```python
from build123d import *

# Parameters (mm, degrees)
BOSS_EXTRUDE1_DEPTH        = 15
FILLET1_R                  = 30
SKETCH4_R                  = 10
CUT_EXTRUDE1_DEPTH         = 5
M10_CLEARANCE_HOLE1_D      = 11
SKETCH7_R                  = 19.05
CUT_EXTRUDE2_DEPTH         = 16
M4_TAPPED_HOLE1_D          = 3.3
CIRPATTERN2_COUNT          = 3
CIRPATTERN3_COUNT          = 3
M12_CLEARANCE_HOLE1_D      = 13
CIRPATTERN4_COUNT          = 3
F_15_0_15_DIAMETER_HOLE1_D = 15
CIRPATTERN5_COUNT          = 3
F_15_0_15_DIAMETER_HOLE2_D = 15
F_9_0_9_DIAMETER_HOLE1_D   = 9


with BuildPart() as part:
    # Sketch1 → Boss-Extrude1 (new body)
    with BuildSketch(Plane(origin=(0, 0, 0), x_dir=(1, 0, 0), z_dir=(0, 1, 0))):
        with BuildLine():
            ThreePointArc((45, 163.935963108), (0, 170), (-45, 163.935963108))
            Line((-45, 163.935963108), (-45, 77.942286341))
            ThreePointArc((-45, 77.942286341), (-77.942286341, 45), (-90, 0))
            Line((-90, 0), (-164.472708645, -42.996838383))
            ThreePointArc((-164.472708645, -42.996838383), (-147.224318643, -85), (-119.472708645, -120.939124724))
            Line((-119.472708645, -120.939124724), (-45, -77.942286341))
            ThreePointArc((-45, -77.942286341), (0, -90), (45, -77.942286341))
            Line((45, -77.942286341), (119.472708645, -120.939124724))
            ThreePointArc((119.472708645, -120.939124724), (147.224318643, -85), (164.472708645, -42.996838383))
            Line((164.472708645, -42.996838383), (90, 0))
            ThreePointArc((90, 0), (77.942286341, 45), (45, 77.942286341))
            Line((45, 77.942286341), (45, 163.935963108))
        make_face()
    extrude(amount=BOSS_EXTRUDE1_DEPTH)

    # Fillet1
    fillet1_edges = [part.edges().sort_by_distance(p)[0] for p in [
        (-119.472708645, 7.5, 120.939124724),
        (-164.472708645, 7.5, 42.996838383),
        (-90, 7.5, 0),
        (-45, 7.5, -77.942286341),
        (-45, 7.5, -163.935963108),
        (45, 7.5, -163.935963108),
        (45, 7.5, -77.942286341),
        (90, 7.5, 0),
        (164.472708645, 7.5, 42.996838383),
        (119.472708645, 7.5, 120.939124724),
        (45, 7.5, 77.942286341),
        (-45, 7.5, 77.942286341),
    ]]
    fillet(fillet1_edges, radius=FILLET1_R)

    # Sketch4 → Cut-Extrude1 (cut)
    with BuildSketch(Plane(origin=(0, 15, 0), x_dir=(1, 0, 0), z_dir=(0, 1, 0))):
        with Locations((0, 148.5)):
            Circle(SKETCH4_R)
    cut_extrude1 = extrude(amount=-CUT_EXTRUDE1_DEPTH, mode=Mode.SUBTRACT)

    # M10 Clearance Hole1 (through all)
    with Locations(Plane(origin=(0, 15, 0), x_dir=(-1, 0, 0), z_dir=(0, 1, 0))):
        with Locations((0, -148.5)):
            m10_clearance_hole1 = Hole(M10_CLEARANCE_HOLE1_D / 2)

    # Sketch7 → Cut-Extrude2 (cut, through all)
    with BuildSketch(Plane(origin=(0, 15, 0), x_dir=(1, 0, 0), z_dir=(0, 1, 0))):
        with Locations((0, 80)):
            Circle(SKETCH7_R)
    cut_extrude2 = extrude(amount=-CUT_EXTRUDE2_DEPTH, mode=Mode.SUBTRACT)

    # M4 Tapped Hole1 (through all)
    with Locations(Plane(origin=(0, 15, 0), x_dir=(1, 0, 0), z_dir=(0, 1, 0))):
        with Locations((-23.57, 103.57), (23.57, 56.43), (23.57, 103.57), (-23.57, 56.43)):
            m4_tapped_hole1 = Hole(M4_TAPPED_HOLE1_D / 2)

    # CirPattern2: Cut-Extrude2, M4 Tapped Hole1 ×3 about axis
    cirpattern2_axis = Axis((0, 0, 0), (0, 1, 0))
    for i in range(1, CIRPATTERN2_COUNT):
        add(cut_extrude2.rotate(cirpattern2_axis, i * 360 / CIRPATTERN2_COUNT), mode=Mode.SUBTRACT)
        add(m4_tapped_hole1.rotate(cirpattern2_axis, i * 360 / CIRPATTERN2_COUNT), mode=Mode.SUBTRACT)

    # CirPattern3: Cut-Extrude1, M10 Clearance Hole1 ×3 about axis
    cirpattern3_axis = Axis((0, 0, 0), (0, 1, 0))
    for i in range(1, CIRPATTERN3_COUNT):
        add(cut_extrude1.rotate(cirpattern3_axis, i * 360 / CIRPATTERN3_COUNT), mode=Mode.SUBTRACT)
        add(m10_clearance_hole1.rotate(cirpattern3_axis, i * 360 / CIRPATTERN3_COUNT), mode=Mode.SUBTRACT)

    # M12 Clearance Hole1 (through all)
    with Locations(Plane(origin=(0, 15, 0), x_dir=(1, 0, 0), z_dir=(0, 1, 0))):
        with Locations((-39.17442065, -65.983537492)):
            m12_clearance_hole1 = Hole(M12_CLEARANCE_HOLE1_D / 2)

    # CirPattern4: M12 Clearance Hole1 ×3 about axis
    cirpattern4_axis = Axis((0, 0, 0), (0, 1, 0))
    for i in range(1, CIRPATTERN4_COUNT):
        add(m12_clearance_hole1.rotate(cirpattern4_axis, i * 360 / CIRPATTERN4_COUNT), mode=Mode.SUBTRACT)

    # Ø15.0 (15) Diameter Hole1 (through all)
    with Locations(Plane(origin=(0, 0, 0), x_dir=(-1, 0, 0), z_dir=(0, -1, 0))):
        with Locations((0, -70)):
            f_15_0_15_diameter_hole1 = Hole(F_15_0_15_DIAMETER_HOLE1_D / 2)

    # CirPattern5: Ø15.0 (15) Diameter Hole1 ×3 about axis
    cirpattern5_axis = Axis((0, 0, 0), (0, 1, 0))
    for i in range(1, CIRPATTERN5_COUNT):
        add(f_15_0_15_diameter_hole1.rotate(cirpattern5_axis, i * 360 / CIRPATTERN5_COUNT), mode=Mode.SUBTRACT)

    # Ø15.0 (15) Diameter Hole2 (through all)
    with Locations(Plane(origin=(0, 0, 0), x_dir=(-1, 0, 0), z_dir=(0, -1, 0))):
        with Locations((0, 0)):
            Hole(F_15_0_15_DIAMETER_HOLE2_D / 2)

    # Ø9.0 (9) Diameter Hole1 (through all)
    with Locations(Plane(origin=(0, 0, 0), x_dir=(-1, 0, 0), z_dir=(0, -1, 0))):
        with Locations((34.641016151, -20)):
            Hole(F_9_0_9_DIAMETER_HOLE1_D / 2)


solid = part.part
```
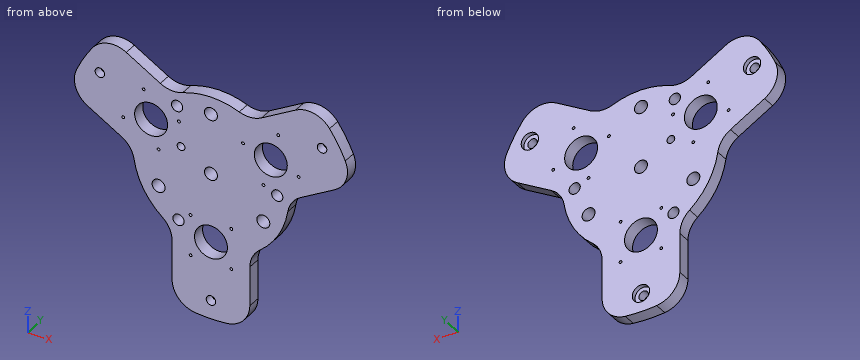
Can you work these out from the model? Positions are in its coordinate system, mm. Coordinates: 2 decimals unless noted, no trailing zeros. Loops run counter-clockwise (first coordinate to the right, second up) from the corner with the lowest first, then second, coordinate; pieces in that order, holes last. Notation, with made-up numbers: (-27, 24.25) - (23, 24.25) arc R14 cw to (23, 42.25) - close; hole circle Ø8 at (41, 60). An arc over 180 degrees is marked (long way). Use a Markdown table: item, result.
Item 1: If I drill on probe 1 along Z at (x, y) = (0, 5); probe 2 along X at (y, z) = (11.5, -39); probe 3 along X at (y, z) = (11.25, 40.5), over which ranges is the centre line in solid material (lowest first)? Write a range as from..to.
Numbers:
| item | result |
|---|---|
| probe 1 | z = -170..-154, -143..-99.05, -60.95..-7.5, 7.5..62.5, 77.5..90 |
| probe 2 | x = -81.11..-66.97, -54.28..54.28, 66.97..81.11 |
| probe 3 | x = -153.36..-88.33, -50.24..50.24, 88.33..153.36 |
Item 2: Will these pins go through, and if not, where does the flat tip stop? pin 1 (7.5 mm diameter, centred on y = 10, z = -109.5, fed in from +X); pin 2 (5 mm diameter, centred on y = 5.5, z = -135.5, fed in from -X); pin 3 (18 mm diameter, centred on x = 0, z = -148.5, fed in from +Y).
Numbers:
| item | result |
|---|---|
| pin 1 | stops at x = 45 |
| pin 2 | stops at x = -45 |
| pin 3 | stops at y = 10 |
Item 3: I want a section at B-B on z = -80. Please give me the cut outline in (x, y).
Numbers:
| item | result |
|---|---|
| outline | (-48.3, 0) - (-19.05, 0) - (-19.05, 15) - (-48.3, 15) - close; (19.05, 0) - (48.3, 0) - (48.3, 15) - (19.05, 15) - close |
Item 4: I want a section at C-C on z = -35. Please give me the cut outline in (x, y), and give its area (3 significant figures).
Numbers:
| item | result |
|---|---|
| outline | (-82.92, 0) - (-68.12, 0) - (-68.12, 15) - (-82.92, 15) - close; (-53.12, 0) - (53.12, 0) - (53.12, 15) - (-53.12, 15) - close; (68.12, 0) - (82.92, 0) - (82.92, 15) - (68.12, 15) - close |
| area | 2,040 mm2 |
Item 5: I want a section at A-A on x = 0. Please give me the cut outline in (y, z), and give its area (3 significant figures).
Numbers:
| item | result |
|---|---|
| outline | (0, -170) - (15, -170) - (15, -158.5) - (10, -158.5) - (10, -154) - (0, -154) - close; (0, -143) - (10, -143) - (10, -138.5) - (15, -138.5) - (15, -99.05) - (0, -99.05) - close; (0, -60.95) - (15, -60.95) - (15, -7.5) - (0, -7.5) - close; (0, 7.5) - (15, 7.5) - (15, 62.5) - (0, 62.5) - close; (0, 77.5) - (15, 77.5) - (15, 90) - (0, 90) - close |
| area | 2,670 mm2 |
Item 6: I want a section at D-D on y = 5.5. Give the number of separate pieces and of enclosed holes in the cut face, and give its area (3 significant figures).
Numbers:
| item | result |
|---|---|
| separate pieces | 1 |
| enclosed holes | 26 |
| area | 42,000 mm2 |
